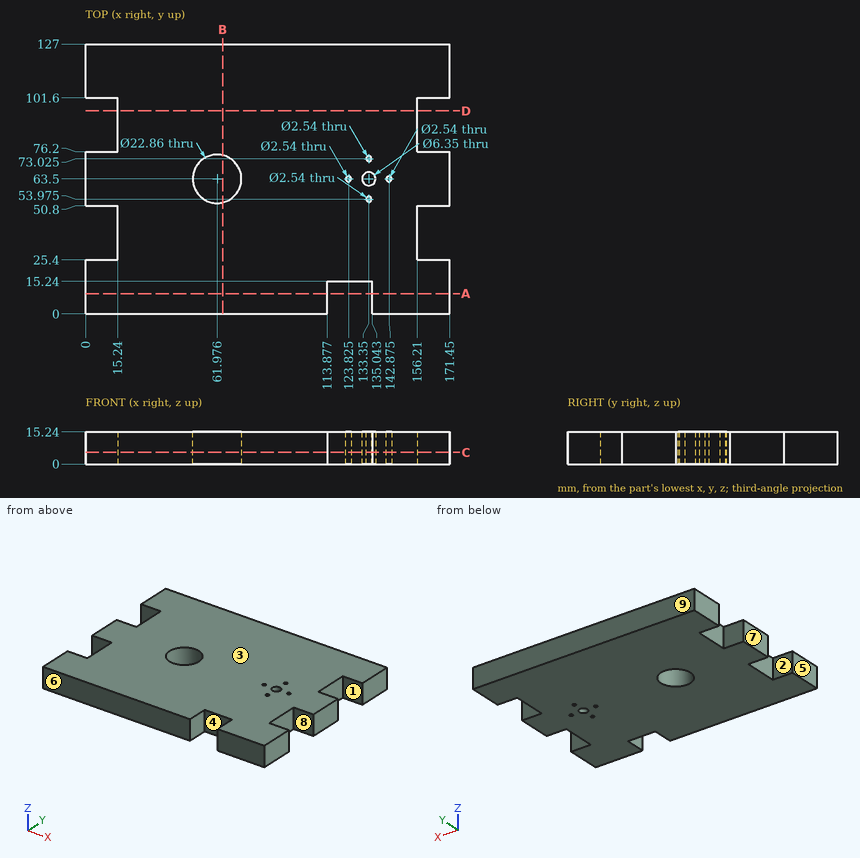
Answer from the drawing. Dimensions are ordinates in mm from the lowest x, y and z of the part. A direction names the side the tool comes from. Round coordinates to 2 decimals unless told otherwise and drop trailing zeros. Loops run counter-clockwise (first coordinate to the right, second up) from the corner with the lowest first, then second, coordinate; pieces in that order, holes last.
(1) For the marked faces 1, 2, 3, 4 and 5, determine the directions among +Z, -Z, +X, -X, +Y, -Y from which every point of the face is accessible in a straight line to the end or side of a thin tool.
Computed values:
face 1: +Z, -Z, +X
face 2: +Z, -Z, -X
face 3: +Z, +X, -X, +Y, -Y
face 4: +Z, -Z, -Y
face 5: +Z, -Z, -X, +Y, -Y
(2) The mould has two halves that part along Y. Classify the marked faces 6, 7, 8 and 9: pulls with the +Y half, pulls with the -Y half, needs draft (parallel to the pull), parting line crosses it, or undercut.
Computed values:
face 6: pulls with the -Y half
face 7: needs draft
face 8: undercut
face 9: pulls with the +Y half
(3) The part is cut by section A-A, the plane y = 9.5. Give the vertices of the cut face in (x, z), and give its area (3 significant figures).
Computed values:
outline: (0, 0) - (113.88, 0) - (113.88, 15.24) - (0, 15.24) - close; (135.04, 0) - (171.45, 0) - (171.45, 15.24) - (135.04, 15.24) - close
area: 2,290 mm2
(4) Each of these flat-tipped pins is pushed along its axis until it touches: P1, Ø1.5, axis at x = 123.825, y = 63.5, coming from the +Z side; P2, Ø12, axis at x = 55.5, y = 86.5, coming from the -Z side; P3, Ø7.5, axis at y = 42, z = 11, coming from the -X side; P4, Ø4.5, axis at y = 32, z = 7.5, coming from the +X side. Where does it stop, or does it pass through?
Computed values:
P1: passes through
P2: stops at z = 0
P3: stops at x = 15.24
P4: stops at x = 156.21
(5) Find the intervals of material crossed by L1, parallel to Y at x = 8.5, z = 4.25; L2, parallel to Y at x = 133.35, z = 10 (1 decimal); L3, parallel to X at y = 11, z = 14, in increasing order.
Computed values:
L1: y = 0 to 25.4, 50.8 to 76.2, 101.6 to 127
L2: y = 15.2 to 52.7, 55.2 to 60.3, 66.7 to 71.8, 74.3 to 127
L3: x = 0 to 113.88, 135.04 to 171.45
(6) The part is cut by section C-C, the plane z = 5.5. Give the number of separate pieces and of enclosed holes in the cut face, and give its area (3 significant figures).
Computed values:
separate pieces: 1
enclosed holes: 6
area: 19,400 mm2
(7) The part is cut by section B-B, the plane x = 64.5. Give the vertices of the cut face in (y, z).
Computed values:
outline: (0, 0) - (52.35, 0) - (52.35, 15.24) - (0, 15.24) - close; (74.65, 0) - (127, 0) - (127, 15.24) - (74.65, 15.24) - close
(8) The part is cut by section D-D, the plane y = 95.5. Give the vertices of the cut face in (x, z), and give its area (3 significant figures).
Computed values:
outline: (15.24, 0) - (156.21, 0) - (156.21, 15.24) - (15.24, 15.24) - close
area: 2,150 mm2
